Verification items for the finished model (mm, model axes). A direction names the side the tool comes from. Round coordinates to 2 decimals unless told otherwise and drop trailing zeros. Write each loop counter-clockwise with the first axis right and the second up, starting at its lowest first coordinate (ties: lowest second). Pieces come first, ordered by that corner, then holes. Notation, with made-up numbers: M 30.25,78.5 L 46.25,78.5 A16 ccw 46.25,85.5 Z; hole C 84,61.25 d1. An arc over 180 degrees is marked long. Answer in a Markdown table with one row per item. Add a question column.
1. Sectioned sample at A-A on z = 0. Record the cut outline in (x, y), plus the area to 3 significant figures.
2. Go/stop test with flat-tipped pins: pin 1 Ø7.5 at (x, z) = (0, 0) entering from +Y; pin 2 Ø3 at (x, y) = (-3.5, 7) entering from +Z; pin 3 Ø4 at (x, y) = (-3, 2.5) entering from -Z. Record where each tip stops, or that it passes through.
3. Draft check along X on faces 1 (the cylindrical face through (-3.86, 4.06, -5.04)), 2 (the flat face through (-7, 0, 0)), 3 (the cylindrical face through (-9.76, 12.32, -2.17)), 4 (the flat face through (0, 17, 0)). Enter one of: pulls with the +X half, pulls with the -X half, needs draft (parallel to the pull), parting line crosses it, or undercut.
4. Set-up check for faces 5 (the cylindrical face through (13.4, 16.89, -0.98)), 6 (the cylindrical face through (-3.86, 21.06, -5.04)), 7 (the flat face through (0, 8, 0)), 8 (the flat face through (-7, 25, 0)): record each of +Z, -Z, +X, -X, +Y, -Y from which the full face is reachable in a straight line by a thin tool's end or side.
5. Sectioned sample at B-B on x = 0. Record the cut outline in (y, z).
6. Material ranges on probe 1 along X at (y, z) = (4.5, 0); probe 2 along Y at (x, z) = (-2.5, 2); probe 3 along Z at (x, y) = (-7.25, 4.5), recorded low to high.
7. Sectioned sample at D-D on z = 6. Record the cut outline in (x, y).
8. Sectioned sample at C-C on y = 18.75. Record the cut outline in (x, z).
```python
from build123d import *

# Parameters (mm, degrees)
SKETCH2_R           = 10
BOSS_EXTRUDE1_DEPTH = 25
SKETCH3_R           = 4.5
BOSS_EXTRUDE2_DEPTH = 18
SKETCH7_R           = 6.35
CUT_EXTRUDE2_DEPTH  = 33.388269645
SKETCH8_W           = 15
SKETCH8_H           = 9
BOSS_EXTRUDE3_DEPTH = 6.5


with BuildPart() as part:
    # Sketch2 → Boss-Extrude1 (new body)
    with BuildSketch(Plane(origin=(0, 0, 0), x_dir=(1, 0, 0), z_dir=(0, 1, 0))):
        with Locations(Location((0, 0, 0), (0, 0, 270))):
            Circle(SKETCH2_R)
    extrude(amount=BOSS_EXTRUDE1_DEPTH)

    # Sketch3 → Boss-Extrude2 (add)
    with BuildSketch(Plane(origin=(0, 0, 0), x_dir=(0, 0, -1), z_dir=(1, 0, 0))):
        with Locations(Location((0, 12.5, 0), (0, 0, 180))):
            Circle(SKETCH3_R)
    extrude(amount=BOSS_EXTRUDE2_DEPTH)

    # Sketch7 → Cut-Extrude2 (cut, through all)
    with BuildSketch(Plane(origin=(0, 25, 0), x_dir=(1, 0, 0), z_dir=(0, 1, 0))):
        with Locations(Location((0, 0, 0), (0, 0, 270))):
            Circle(SKETCH7_R)
    extrude(amount=-CUT_EXTRUDE2_DEPTH, mode=Mode.SUBTRACT)

    # Sketch8 → Boss-Extrude3 (add, symmetric)
    with BuildSketch(Plane.XY):
        with Locations((0, 12.5)):
            Rectangle(SKETCH8_W, SKETCH8_H)
    extrude(amount=BOSS_EXTRUDE3_DEPTH, both=True)


solid = part.part
```
Geometry check:
| question | item | result |
|---|---|---|
| 1 | outline | M -10,0 L -6.35,0 L -6.35,8 L 6.35,8 L 6.35,0 L 10,0 L 10,8 L 18,8 L 18,17 L 10,17 L 10,25 L 6.35,25 L 6.35,17 L -6.35,17 L -6.35,25 L -10,25 Z |
| 1 | area | 369 mm2 |
| 2 | pin 1 | stops at y = 17 |
| 2 | pin 2 | stops at z = 9.8 |
| 2 | pin 3 | stops at z = -9.95 |
| 3 | face 1 | undercut |
| 3 | face 2 | needs draft |
| 3 | face 3 | parting line crosses it |
| 3 | face 4 | undercut |
| 4 | face 5 | +X |
| 4 | face 6 | +Y |
| 4 | face 7 | -Y |
| 4 | face 8 | +Z, -Z, +X, -X, +Y |
| 5 | outline | M 0,-10 L 25,-10 L 25,-6.35 L 17,-6.35 L 17,6.35 L 25,6.35 L 25,10 L 0,10 L 0,6.35 L 8,6.35 L 8,-6.35 L 0,-6.35 Z |
| 6 | probe 1 | x = -10 to -6.35, 6.35 to 10 |
| 6 | probe 2 | y = 8 to 17 |
| 6 | probe 3 | z = -6.89 to 6.89 |
| 7 | outline | M -8,0 L -2.08,0 L -2.08,8 L 2.08,8 L 2.08,0 L 8,0 L 8,25 L 2.08,25 L 2.08,17 L -2.08,17 L -2.08,25 L -8,25 Z |
| 8 | outline | C 0,0 d20; hole C 0,0 d12.7 |
